Check sheet for the modelled part. Datum: model origin and axes. Units: mm. A direction names the side the tool comes from. Give positions to 0.01 mm unless a question says otherwise; leave off trailing zeros. Write each loop counter-clockwise with the first axis right and the second up, starting at its lowest first coordinate (ties: lowest second). Pieces come first, ordered by that corner, then holes. Notation, with made-up numbers: (48.5, 88.25) - (105.5, 88.25) arc R26 ccw to (105.5, 115.25) - close; hole circle Ø3 at (85.25, -18). An arc over 180 degrees is marked (long way). Return JSON: item names as keys, results as strings. Group by question number.
Autodesk Inventor part; units mm, degrees
ref_plane "YZ Plane" through (0, 0, 0) normal (1, 0, 0) x (0, 1, 0)
ref_plane "XZ Plane" through (0, 0, 0) normal (0, 1, 0) x (-1, 0, 0)
ref_plane "XY Plane" through (0, 0, 0) normal (0, 0, 1) x (1, 0, 0)
ref_plane "Work Plane2" through (0, 0, 0) normal (0, 0, 1) x (1, 0, 0)
sketch "Sketch3" plane through (0, 0, 0) normal (0, 0, 1) x (1, 0, 0)
  line L0 (-24.13, 20.32) -> (-25.146, 20.32)
  arc A0 (-25.146, 20.32) -> (-31.75, 13.716) centre (-25.146, 13.716) ccw
  line L1 (-31.75, 13.716) -> (-31.75, 6.096)
  arc A1 (-25.146, 12.7) -> (-31.75, 6.096) centre (-25.146, 6.096) ccw
  line L2 (-24.13, 12.7) -> (-25.146, 12.7)
  line L3 (-24.13, 20.32) -> (-24.13, 12.7) construction
  circle A2 centre (-27.94, 15.24) radius 1.1303
  line L4 (-24.13, 12.7) -> (-17.13, 12.7)
  line L5 (-17.13, 12.7) -> (-17.13, 20.32)
  line L6 (-17.13, 20.32) -> (-24.13, 20.32)
  line L7 (-24.13, 20.32) -> (-24.13, 20.2414)
  line L8 (-24.13, 12.7) -> (-31.75, 12.7)
  point P0 (0, 0)
  dimension "d0" = 7
extrude "Extrusion1" add sketch "Sketch3" along normal blind 3.175 contours L6 L5 L4 L2 L8 L1 A0 L0
sketch "Sketch4" plane through (0, 0, 0) normal (0, 0, -1) x (-1, 0, 0)
  line L0 (20.13, 20.32) -> (20.13, 12.7) construction
  line L1 (22.13, 12.7) -> (22.13, 20.32) construction
  line L2 (17.13, 20.32) -> (25.146, 20.32)
  line L3 (31.75, 12.7) -> (17.13, 12.7)
  line L4 (20.03, 20.32) -> (18.23, 20.32)
  line L5 (18.23, 20.32) -> (18.23, 12.7)
  line L6 (18.23, 12.7) -> (20.03, 12.7)
  line L7 (20.03, 12.7) -> (20.03, 20.32)
  line L8 (22.23, 20.32) -> (24.03, 20.32)
  line L9 (24.03, 20.32) -> (24.03, 12.7)
  line L10 (24.03, 12.7) -> (22.23, 12.7)
  line L11 (22.23, 12.7) -> (22.23, 20.32)
  line L12 (24.13, 20.32) -> (24.13, 12.7) construction
  point P0 (0, 0)
  dimension "d3" = 0.1
  dimension "d4" = 0.1
  dimension "d6" = 0.1
extrude "Extrusion2" add sketch "Sketch4" along normal blind 6.35 contours L2 L7 L3 L5 | L2 L9 L3 L11
sketch "Sketch5" plane through (-18.23, 12.7, 0) normal (1, 0, 0) x (0, 0, -1)
  line L0 (0, 1.016) -> (0, 0)
  line L1 (6.35, 0) -> (6.35, 7.62)
  line L2 (0, 0) -> (6.35, 7.62) construction
  circle A0 centre (3.175, 3.81) radius 1.5875
  point P0 (0, -12.7)
  dimension "d9" = 3.175
extrude "Extrusion3" cut sketch "Sketch5" against normal blind 9.75
properties part number "adapter2"
Item 1: Material ranges on line 1 along X through (y, z) = (19.75, -0.5); line 2 along Z through (x, y) = (-28.75, 16.5) (3 decimals); line 3 along X through (y, z) = (17.25, 2), recorded low to high. Write a range as from..to.
Item 2: Mould release check, pull along Z, two halves, no side actions. Record for faces 1 (the face through (-25, 17, 3.175)), 2 (the face through (-23.12, 14.96, -2.83)), 3 (the face through (-19.12, 14.96, -2.83)), 4 (the face through (-29.9, 18.3, 1.6)): +Z half, -Z half, draft (parallel to the pull), parting line (faces both ways), or undercut.
Item 3: Section check C-C on y = 16.75. Record the cut outline in (x, z) (3 decimals), plus the area to 3 significant figures.
Item 4: Section check A-A on x = -27.94. Record the cut outline in (y, z) (3 decimals), plus the area to 3 significant figures.
Item 5: Section check D-D on y = 13.5. Record the cut outline in (x, z) (3 decimals).
Item 6: Section check B-B on z = -3. Record the cut outline in (x, y).
Item 7: Access from +Z, -Z, +X, -X, +Y, -Y to the whole of each face (thin tool, end or side, straight path). Record for faces 5 (the face through (-27, 17, 0)), 6 (the face through (-19, 17, -6.35)), 7 (the face through (-20.03, 16, -5)), 8 (the face through (-18, 17, 0)), 9 (the face through (-28.837, 15.928, 1.565)).
Item 8: Depth check by flat-ended pin: pin 1 (2.5 mm diameter, centred on y = 16.51, z = -3.175, fed in from -X); pin 2 (3 mm diameter, centred on y = 15.5, z = -4, fed in from +X); pin 3 (1.2 mm diameter, centred on x = -17.5, y = 15.5, fed in from -Z). Enter the tip coordinate at first touch or a pass-through.
Reply:
{
 "1": {"line 1": "-24.03..-22.23, -20.03..-18.23", "line 2": "0..3.175", "line 3": "-30.72..-17.13"},
 "2": {"face 1": "+Z half", "face 2": "undercut", "face 3": "undercut", "face 4": "draft"},
 "3": {"outline": "(-31.012, 0) - (-24.03, 0) - (-24.03, -1.606) - (-22.23, -1.606) - (-22.23, 0) - (-20.03, 0) - (-20.03, -1.606) - (-18.23, -1.606) - (-18.23, 0) - (-17.13, 0) - (-17.13, 3.175) - (-31.012, 3.175) - close; (-24.03, -6.35) - (-22.23, -6.35) - (-22.23, -4.744) - (-24.03, -4.744) - close; (-20.03, -6.35) - (-18.23, -6.35) - (-18.23, -4.744) - (-20.03, -4.744) - close", "area": "55.6 mm²"},
 "4": {"outline": "(12.7, 0) - (14.11, 0) - (14.11, 3.175) - (12.7, 3.175) - close; (16.37, 0) - (19.7, 0) - (19.7, 3.175) - (16.37, 3.175) - close", "area": "15.0 mm²"},
 "5": {"outline": "(-31.75, 0) - (-24.03, 0) - (-24.03, -6.35) - (-22.23, -6.35) - (-22.23, 0) - (-20.03, 0) - (-20.03, -6.35) - (-18.23, -6.35) - (-18.23, 0) - (-17.13, 0) - (-17.13, 3.175) - (-31.75, 3.175) - close"},
 "6": {"outline": "(-24.03, 12.7) - (-22.23, 12.7) - (-22.23, 14.93) - (-24.03, 14.93) - close; (-24.03, 18.09) - (-22.23, 18.09) - (-22.23, 20.32) - (-24.03, 20.32) - close; (-20.03, 12.7) - (-18.23, 12.7) - (-18.23, 14.93) - (-20.03, 14.93) - close; (-20.03, 18.09) - (-18.23, 18.09) - (-18.23, 20.32) - (-20.03, 20.32) - close"},
 "7": {"face 5": "-Z, -X, +Y, -Y", "face 6": "-Z, +X, -X, +Y, -Y", "face 7": "-Z, +Y, -Y", "face 8": "-Z, +X, +Y, -Y", "face 9": "+Z, -Z"},
 "8": {"pin 1": "through", "pin 2": "x = -18.23", "pin 3": "z = 0"}
}
